CAD build for the part. Positions are in the model's coordinates, mm. Face numbers are marked on the shaded views. A direction names the side the tool comes from. Round coordinates to 2 decimals unless told otherwise and drop trailing zeros. Order: outer loops, then holes, each group sorted by start corner. A loop starts at its lowest first (then second) coordinate and runs counter-clockwise, first axis right, second up. Notation, with made-up numbers: M 43.5,54 L 63.5,54 A31 ccw 63.5,93 Z; hole C -1.75,54 d3. An arc over 180 degrees is marked long. Answer as a JSON object with one key per item and string values.
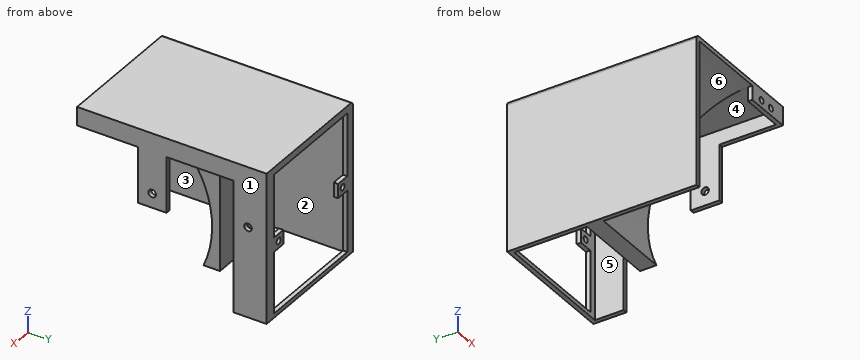
Autodesk Fusion 360 part; units mm, degrees
sketch "스케치1" plane through (0, 0, 0) normal (0, 1, 0) x (1, 0, 0)
  line L0 (-46.5, -52.5) -> (46.5, -52.5)
  line L1 (46.5, -52.5) -> (46.5, 52.5)
  line L2 (46.5, 52.5) -> (-46.5, 52.5)
  line L3 (-46.5, 52.5) -> (-46.5, -52.5)
  line L4 (-46.5, -52.5) -> (46.5, 52.5) construction
  line L5 (46.5, -52.5) -> (-46.5, 52.5) construction
  line L6 (0, -52.5) -> (0, -47.5)
  line L7 (0, 52.5) -> (0, 49.5)
  line L8 (46.5, 0) -> (38.5, 0)
  line L9 (-46.5, 0) -> (-40.5, 0)
  line L10 (-40.5, 0) -> (-40.5, -47.5)
  line L11 (-40.5, -47.5) -> (38.5, -47.5)
  line L12 (38.5, -47.5) -> (38.5, 49.5)
  line L13 (38.5, 49.5) -> (-40.5, 49.5)
  line L14 (-40.5, 49.5) -> (-40.5, 0)
  dimension "d1" = 105
  dimension "d2" = 93
  dimension "d3" = 5
  dimension "d4" = 3
  dimension "d5" = 8
  dimension "d6" = 6
extrude "돌출1" add sketch "스케치1" along normal blind 132.5 contours L0 L3 L6 L9 L10 L11 | L0 L1 L6 L8 L11 L12 | L2 L3 L7 L9 L13 L14 | L1 L2 L7 L8 L12 L13
sketch "스케치2" plane through (0, 0, 0) normal (0, -1, 0) x (1, 0, 0)
  line L0 (-40.5, -49.5) -> (-40.5, 47.5)
  line L1 (-40.5, 47.5) -> (38.5, 47.5)
  line L2 (38.5, 47.5) -> (38.5, -49.5)
  line L3 (38.5, -49.5) -> (-40.5, -49.5)
  line L4 (-46.5, 52.5) -> (-46.5, -52.5)
  line L5 (-46.5, -52.5) -> (46.5, -52.5)
  line L6 (46.5, -52.5) -> (46.5, 52.5)
  line L7 (46.5, 52.5) -> (-46.5, 52.5)
  line L8 (-46.5, 52.5) -> (-43.5, 52.5)
  line L9 (-43.5, 52.5) -> (-43.5, 49.5)
  line L10 (-43.5, 49.5) -> (-46.5, 49.5)
  line L11 (-46.5, 49.5) -> (-46.5, 52.5)
  line L12 (46.5, -52.5) -> (43.5, -52.5)
  line L13 (-43.5, 49.5) -> (43.5, 49.5)
  line L14 (43.5, 49.5) -> (43.5, -52.5)
  line L15 (43.5, -52.5) -> (-43.5, -52.5)
  line L16 (-43.5, -52.5) -> (-43.5, 49.5)
  dimension "d9" = 3
  dimension "d10" = 3
  dimension "d11" = 3
extrude "돌출2" cut sketch "스케치2" against normal blind 129.5 contours L5 L13 L14 L15 L16
sketch "스케치3" plane through (-46.5, 0, 0) normal (-1, 0, 0) x (0, -1, 0)
  line L0 (0, -52.5) -> (0, 52.5)
  line L1 (0, 52.5) -> (-132.5, 52.5)
  line L2 (-132.5, 52.5) -> (-132.5, -52.5)
  line L3 (-132.5, -52.5) -> (0, -52.5)
  line L4 (0, 52.5) -> (0, -23.5)
  circle A0 centre (0, -23.5) radius 73
  circle A1 centre (0, -23.5) radius 75.5
  line L5 (0, 52.5) -> (-42.5, 52.5)
  line L6 (-42.5, 52.5) -> (-42.5, 35.8528)
  line L7 (-42.5, 35.8528) -> (0, 35.8528)
  line L8 (0, 35.8528) -> (0, 52.5)
  line L9 (0, 52.5) -> (-3, 52.5)
  line L10 (-3, 52.5) -> (-3, 49.4383)
  line L11 (-3, 49.4383) -> (0, 49.4383)
  line L12 (0, 49.4383) -> (0, 52.5)
  line L13 (-66.9925, -52.5) -> (-62.9352, -52.5)
  line L14 (-62.9352, -52.5) -> (-62.9352, -49.5)
  line L15 (-62.9352, -49.5) -> (-66.9925, -49.5)
  line L16 (-66.9925, -49.5) -> (-66.9925, -52.5)
  line L17 (0, 52.5) -> (-75.5, 52.5)
  line L18 (-75.5, 52.5) -> (-75.5, -52.5)
  line L19 (-75.5, -52.5) -> (0, -52.5)
  line L20 (0, -52.5) -> (0, 52.5)
  dimension "d14" = 76
  dimension "d15" = 146
  dimension "d16" = 151
  dimension "d45" = 42.5
  dimension "d46" = 3
  dimension "d50" = 3
  dimension "d71" = 75.5
extrude "돌출3" cut sketch "스케치3" against normal blind 10 contours L0 L3 L4 A0 L8 L12 L13 L19 L20
sketch "스케치4" plane through (0, 132.5, 0) normal (0, 1, 0) x (-1, 0, 0)
  line L0 (40.5, 47.5) -> (40.5, -49.5)
  line L1 (40.5, -49.5) -> (-38.5, -49.5)
  line L2 (-38.5, -49.5) -> (-38.5, 47.5)
  line L3 (-38.5, 47.5) -> (40.5, 47.5)
  line L4 (46.5, -52.5) -> (46.5, 52.5)
  line L5 (46.5, 52.5) -> (-46.5, 52.5)
  line L6 (-46.5, 52.5) -> (-46.5, -52.5)
  line L7 (-46.5, -52.5) -> (46.5, -52.5)
  line L8 (-38.5, -49.5) -> (-38.5, -6.5)
  line L9 (-38.5, -6.5) -> (-28.5, -6.5)
  line L10 (-28.5, -6.5) -> (-28.5, 3.5)
  line L11 (-28.5, 3.5) -> (-38.5, 3.5)
  line L12 (-38.5, 3.5) -> (-38.5, -6.5)
  line L13 (40.5, -6.5) -> (30.5, -6.5)
  line L14 (30.5, -6.5) -> (30.5, 3.5)
  line L15 (30.5, 3.5) -> (40.5, 3.5)
  line L16 (40.5, 3.5) -> (40.5, -6.5)
  circle A0 centre (-33.5, -1.5) radius 2.15
  circle A1 centre (35.5, -1.5) radius 2.15
  dimension "d19" = 43
  dimension "d20" = 10
  dimension "d21" = 10
  dimension "d22" = 10
  dimension "d23" = 10
  dimension "d24" = 4.3
  dimension "d25" = 4.3
extrude "돌출4" add sketch "스케치4" against normal blind 3 contours L0 L13 L14 L15 L16 | L2 L9 L10 L11 L12
sketch "스케치5" plane through (43.5, 0, 0) normal (-1, 0, 0) x (0, -1, 0)
  line L0 (0, -52.5) -> (0, 49.5)
  line L1 (0, 49.5) -> (-129.5, 49.5)
  line L2 (-129.5, 49.5) -> (-129.5, -52.5)
  line L3 (-129.5, -52.5) -> (0, -52.5)
  line L4 (-129.5, 49.5) -> (-109.5, 49.5)
  line L5 (-109.5, 49.5) -> (-109.5, -52.5)
  line L6 (-109.5, -52.5) -> (-129.5, -52.5)
  line L7 (-129.5, -52.5) -> (-129.5, 49.5)
  line L8 (-109.5, 49.5) -> (-62.5, 49.5)
  line L9 (-62.5, 49.5) -> (-42.5, 49.5)
  line L10 (-42.5, 49.5) -> (-42.5, -52.5)
  line L11 (-42.5, -52.5) -> (-62.5, -52.5)
  line L12 (-62.5, -52.5) -> (-62.5, 49.5)
  line L13 (-42.5, 49.5) -> (-42.5, 20.5)
  line L14 (-109.5, 20.5) -> (-129.5, 20.5)
  line L15 (-129.5, 20.5) -> (-129.5, 0.5)
  line L16 (-129.5, 0.5) -> (-109.5, 0.5)
  line L17 (-109.5, 0.5) -> (-109.5, 20.5)
  circle A0 centre (-119.5, 10.5) radius 2.65
  line L18 (-42.5, 20.5) -> (-62.5, 20.5)
  line L19 (-62.5, 20.5) -> (-62.5, 0.5)
  line L20 (-62.5, 0.5) -> (-42.5, 0.5)
  line L21 (-42.5, 0.5) -> (-42.5, 20.5)
  circle A1 centre (-52.5, 10.5) radius 2.65
  dimension "d28" = 20
  dimension "d29" = 47
  dimension "d30" = 20
  dimension "d31" = 29
  dimension "d33" = 20
  dimension "d34" = 20
  dimension "d36" = 5.3
  dimension "d41" = 20
  dimension "d42" = 5.3
extrude "돌출5" cut sketch "스케치5" against normal blind 3 contours L0 L1 L3 L10 L13 L21 | L3 L10 L11 L12 L20 | L1 L3 L5 L8 L12 L17 L19 | A0 | A1
extrude "돌출19" add sketch "스케치3" against normal blind 60 contours L3 A0 A1 L6 L19 | A0 A1 L6 L10 | L3 A1 L18 L19 | L0 L4 A0 A1 L8 L10 L12 L20 | L1 A1 L5 L6 L10 L17 | L1 A1 L6 L17 L18 | L0 L1 L4 A1 L5 L8 L9 L10 L12 L17 L20
extrude "돌출21" add 1 faces at (-24.5, 75.5, 15.5) along direction (0, 1, 0) blind 3
sketch "스케치12" plane through (0, 0, 49.5) normal (0, 0, -1) x (1, 0, 0)
  line L0 (13.5, -78.5) -> (-43.5, -78.5)
  line L1 (-43.5, -78.5) -> (-43.5, -129.5)
  line L2 (-43.5, -129.5) -> (43.5, -129.5)
  line L3 (43.5, -129.5) -> (43.5, -109.5)
  line L4 (43.5, -109.5) -> (46.5, -109.5)
  line L5 (46.5, -109.5) -> (46.5, -62.5)
  line L6 (46.5, -62.5) -> (43.5, -62.5)
  line L7 (43.5, -62.5) -> (43.5, -42.5)
  line L8 (43.5, -42.5) -> (46.5, -42.5)
  line L9 (46.5, -42.5) -> (46.5, 0)
  line L10 (46.5, 0) -> (13.5, 0)
  line L11 (13.5, 0) -> (13.5, -78.5)
  line L12 (46.5, 0) -> (13.5, 0)
  line L13 (13.5, 0) -> (13.5, -3)
  line L14 (13.5, -3) -> (46.5, -3)
  line L15 (46.5, -3) -> (46.5, 0)
  line L16 (43.5, -129.5) -> (46.5, -129.5)
  line L17 (46.5, -129.5) -> (46.5, 0)
  line L18 (46.5, 0) -> (43.5, 0)
  line L19 (43.5, 0) -> (43.5, -129.5)
  dimension "d103" = 3
extrude "돌출22" add sketch "스케치12" along normal blind 10 contours L10 L11 L12 L13 L14 L19 | L9 L10 L12 L14 L15 L17 L18 L19 | L8 L9 L14 L17 L19 | L4 L5 L6 L17 L19
sketch "스케치13" plane through (0, 0, 0) normal (0, -1, 0) x (1, 0, 0)
  line L0 (46.5, 39.5) -> (46.5, 52.5)
  line L1 (46.5, 52.5) -> (-46.5, 52.5)
  line L2 (-46.5, 52.5) -> (-46.5, 49.5)
  line L3 (-46.5, 49.5) -> (13.5, 49.5)
  line L4 (13.5, 49.5) -> (13.5, 39.5)
  line L5 (13.5, 39.5) -> (46.5, 39.5)
  line L6 (46.5, 52.5) -> (43.5, 52.5)
  line L7 (43.5, 52.5) -> (43.5, 39.5)
  line L8 (43.5, 39.5) -> (46.5, 39.5)
  line L9 (46.5, 39.5) -> (46.5, 52.5)
  line L10 (13.5, 39.5) -> (43.5, 39.5)
  line L11 (43.5, 39.5) -> (43.5, 49.5)
  line L12 (43.5, 49.5) -> (13.5, 49.5)
  line L13 (13.5, 49.5) -> (13.5, 39.5)
  line L14 (13.5, 44.5) -> (23.5, 44.5)
  line L15 (23.5, 44.5) -> (33.5, 44.5)
  circle A0 centre (23.5, 44.5) radius 2.15
  circle A1 centre (33.5, 44.5) radius 2.15
  dimension "d106" = 3
  dimension "d107" = 10
  dimension "d108" = 10
  dimension "d109" = 10
  dimension "d110" = 4.3
  dimension "d111" = 4.3
extrude "돌출23" cut sketch "스케치13" against normal blind 3 contours A1 | L14 L15 A0 | L14 L15 A0
fillet "필렛2" radius 2.5 1 edges at (-46.5, 66.25, 52.5)
Item 1: Two-plate mould, pull along Y, no slides. Class the marked faces 3, 4, 5 and 6: released by +Y, released by -Y, zero draft, split by the parting line, or undercut.
Worked answers:
{"face 3": "zero draft", "face 4": "undercut", "face 5": "undercut", "face 6": "released by -Y"}
Item 2: Saw through at C-C on z = -1.5. List the corners of the cut face in (x, y).
Worked answers:
{"outline": "M -46.5,0 L -43.5,0 L -43.5,69.61 L 13.5,69.61 L 13.5,78.5 L -43.5,78.5 L -43.5,129.5 L -37.65,129.5 L -37.65,132.5 L -46.5,132.5 Z; M -33.35,129.5 L -30.5,129.5 L -30.5,132.5 L -33.35,132.5 Z; M 28.5,129.5 L 31.35,129.5 L 31.35,132.5 L 28.5,132.5 Z; M 35.65,129.5 L 43.5,129.5 L 43.5,109.5 L 46.5,109.5 L 46.5,132.5 L 35.65,132.5 Z"}
Item 3: 3-axis set-ups, long thin cutter, end or side, ignore diameter. For the marked faces 1 and 2: which of +Z, -Z, +X, -X, +Y, -Y reach the whole face in a straight line?
Worked answers:
{"face 1": "+Z, -Z, +X, +Y, -Y", "face 2": "-Z"}
Item 4: Saw through at A-A on y = 119.5. List the corners of the cut face in (x, z).
Worked answers:
{"outline": "M -46.5,-52.5 L -43.5,-52.5 L -43.5,49.5 L 43.5,49.5 L 43.5,13.15 L 46.5,13.15 L 46.5,52.5 L -44,52.5 A2.5 ccw -46.5,50 Z; M 43.5,-52.5 L 46.5,-52.5 L 46.5,7.85 L 43.5,7.85 Z"}
Item 5: Wall check: line 1 along Z through (x, y) = (33.5, 131); line 2 along X through (y, z) = (2.25, 44.5); line 3 along Z through (x, y) = (33.5, 1.5). Give the ranges that are in metal, low to high. Write a range as [from, to].
Worked answers:
{"line 1": "z = [-52.5, -49.5], [-6.5, -3.65], [0.65, 3.5], [47.5, 52.5]", "line 2": "x = [-46.5, -43.5], [13.5, 21.35], [25.65, 31.35], [35.65, 46.5]", "line 3": "z = [39.5, 42.35], [46.65, 52.5]"}
Item 6: Drop flat-ended pins along their axis: pin 1 Ø12 at (y, z) = (69, -4) entering from +X; pin 2 Ø2 at (x, z) = (-18, 4.5) entering from -Y; pin 3 Ø4 at (x, y) = (-17, 84) entering from -Z. Give the stop position or say it passes through.
Worked answers:
{"pin 1": "stops at x = 13.5", "pin 2": "stops at y = 66.99", "pin 3": "stops at z = 49.5"}
Item 7: Saw through at D-D on x = 33.5. List the corners of the cut face in (y, z).
Worked answers:
{"outline": "M 0,39.5 L 3,39.5 L 3,42.35 L 0,42.35 Z; M 0,46.65 L 3,46.65 L 3,49.5 L 129.5,49.5 L 129.5,47.5 L 132.5,47.5 L 132.5,52.5 L 0,52.5 Z; M 129.5,-52.5 L 132.5,-52.5 L 132.5,-49.5 L 129.5,-49.5 Z; M 129.5,-6.5 L 132.5,-6.5 L 132.5,-3.65 L 129.5,-3.65 Z; M 129.5,0.65 L 132.5,0.65 L 132.5,3.5 L 129.5,3.5 Z"}
Item 8: Saw through at B-B on x = 23.5. List the corners of the cut face in (y, z).
Worked answers:
{"outline": "M 0,39.5 L 3,39.5 L 3,42.35 L 0,42.35 Z; M 0,46.65 L 3,46.65 L 3,49.5 L 129.5,49.5 L 129.5,47.5 L 132.5,47.5 L 132.5,52.5 L 0,52.5 Z; M 129.5,-52.5 L 132.5,-52.5 L 132.5,-49.5 L 129.5,-49.5 Z"}
